Geometry: see drawing. Coordinates: mm, zero at the bounding-box minimum. A direction names the side the tool comes from. Give positions to 0.01 mm unless a question says otherwise; leave off trailing zeros. Write each loop counter-clockwise with the first axis right and the second up, starting at its lowest first coordinate (ties: lowest second). Pieces come first, ordered by that corner, then holes. Notation, with made-up numbers: (89.5, -38.5) - (133.5, -38.5) arc R11 cw to (133.5, -19.5) - close; hole circle Ø3 at (32.5, 38). An arc over 180 degrees is marked (long way). Answer as CSV lines item,"result". Start each with the question number.
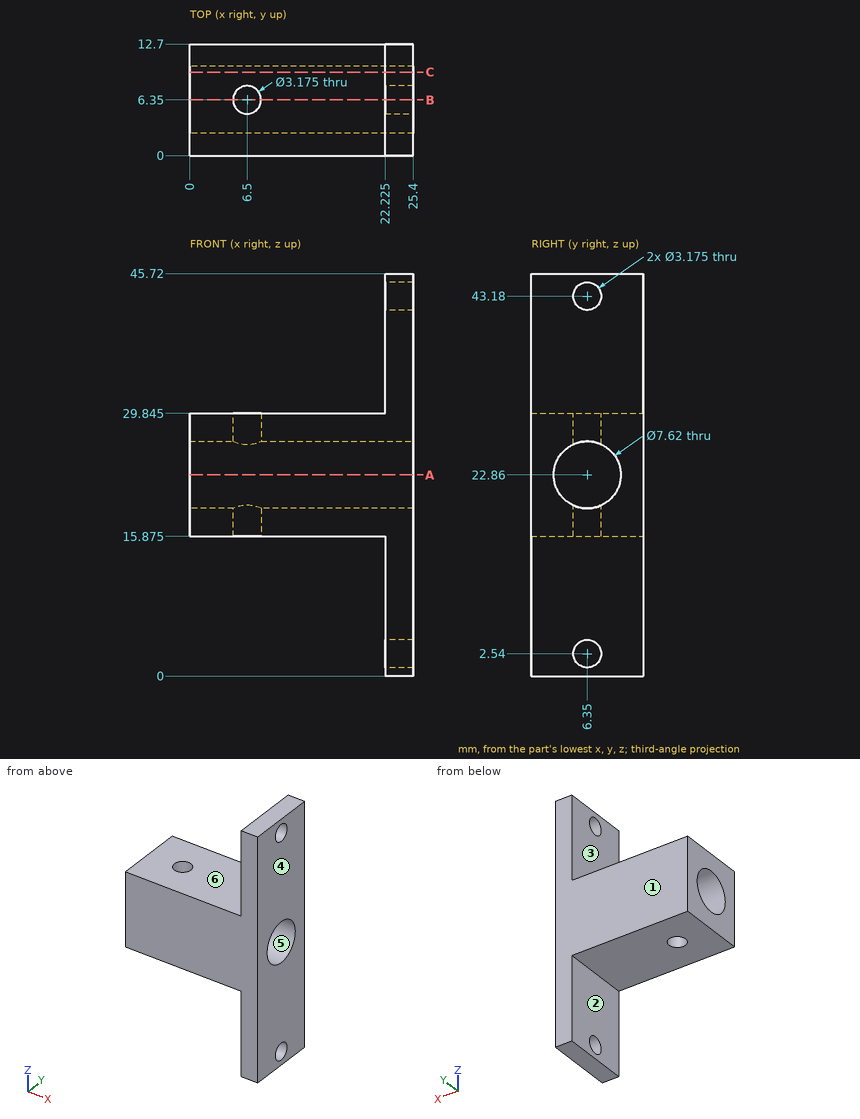
1) Material intervals for line 1 (Y direction, x = 18.5, z = 22.86); line 2 (X direction, y = 2.5, z = 34) (1 decimal); line 3 (Z direction, x = 9.5, y = 6.5) (1 decimal), sorted ascending. Write a range as from..to.
2) Cut plane B-B on y = 6.35. State how many separate pieces and enclosed holes the cut face has, and give its area (3 significant figures).
3) Reachability of the marked faces 1, 2 and 3 from +Z, -Z, +X, -X, +Y, -Y: full face, straight path, thin tool, end or side. Return the list, or none.
4) Contact query for flat-ended pins moving along their axis: P1, Ø8, axis at x = 14.5, z = 24, coming from the -Y side; P2, Ø5, axis at x = 6.5, y = 6.35, coming from the -Z side (3 decimals); P3, Ø3, axis at y = 5, z = 6.5, coming from the -X side (3 decimals); P4, Ø6.5, axis at x = 8, y = 8.5, coming from the +Z side (3 decimals). Output: stop coordinate, or through.
5) Pull-direction query (Z, two-part tool) for the marked faces 4, 5 and 6; classes: +Z half, -Z half, draft (parallel to the pull), parting line (faces both ways), or undercut.
6) Cut plane A-A on z = 22.86. Output: boundary loops of the cut face in (x, y), and give its area (3 significant figures).
7) Cut plane C-C on y = 9.5. Output: boundary loops of the cut face in (x, z) (1 decimal).
Numbers:
1,line 1,"y = 0..2.54, 10.16..12.7"
1,line 2,"x = 22.2..25.4"
1,line 3,"z = 15.9..19.1, 26.7..29.8"
2,separate pieces,"6"
2,enclosed holes,"0"
2,area,"222 mm²"
3,face 1,"+Z, -Z, +X, -X, +Y"
3,face 2,"-Z, -X, +Y, -Y"
3,face 3,"+Z, -X, +Y, -Y"
4,P1,"stops at y = 0"
4,P2,"stops at z = 15.875"
4,P3,"stops at x = 22.225"
4,P4,"stops at z = 29.845"
5,face 4,"draft"
5,face 5,"undercut"
5,face 6,"+Z half"
6,outline,"(0, 0) - (25.4, 0) - (25.4, 2.54) - (0, 2.54) - close; (0, 10.16) - (25.4, 10.16) - (25.4, 12.7) - (0, 12.7) - close"
6,area,"129 mm²"
7,outline,"(0, 15.9) - (22.2, 15.9) - (22.2, 0) - (25.4, 0) - (25.4, 20.7) - (0, 20.7) - close; (0, 25) - (25.4, 25) - (25.4, 45.7) - (22.2, 45.7) - (22.2, 29.8) - (0, 29.8) - close"
